from build123d import *

# Parameters (mm, degrees)
SKETCH2_W                      = 25.4
SKETCH2_H                      = 50.8
SKETCH2_W_2                    = 22.225
SKETCH2_H_2                    = 47.625
EXTRUDE_THIN2_DEPTH            = 1828.8
CUT_EXTRUDE1_DEPTH             = 26.4
F_9_16_0_5625_DIAMETER_HOLE1_D = 14.2875
F_9_16_0_5625_DIAMETER_HOLE2_D = 14.2875
F_12_0MM_DOWEL_HOLE1_D         = 12
F_3_16_0_1875_DIAMETER_HOLE1_D = 4.7625


with BuildPart() as part:
    # Sketch2 → Extrude-Thin2 (new body)
    with BuildSketch(Plane.XY):
        Rectangle(SKETCH2_W, SKETCH2_H)
        Rectangle(SKETCH2_W_2, SKETCH2_H_2, mode=Mode.SUBTRACT)
    extrude(amount=EXTRUDE_THIN2_DEPTH)

    # Sketch8 → Cut-Extrude1 (cut, through all)
    with BuildSketch(Plane(origin=(12.7, 0, 0), x_dir=(0, 0, -1), z_dir=(1, 0, 0))):
        with BuildLine():
            Line((-1828.8, 25.4), (-1828.8, -3.09e-07))
            ThreePointArc((-1828.8, -3.09e-07), (-1824.623790622, 14.87379041), (-1813.315860361, 25.4))
            Line((-1813.315860361, 25.4), (-1828.8, 25.4))
        make_face()
        with BuildLine():
            Line((-1828.8, -25.4), (-1813.315860361, -25.4))
            ThreePointArc((-1813.315860361, -25.4), (-1824.623790462, -14.873790674), (-1828.8, -3.09e-07))
            Line((-1828.8, -3.09e-07), (-1828.8, -25.4))
        make_face()
    extrude(amount=-CUT_EXTRUDE1_DEPTH, mode=Mode.SUBTRACT)

    # 9/16 (0.5625) Diameter Hole1 (through all)
    with Locations(Plane(origin=(12.7, 0, 0), x_dir=(0, 0, -1), z_dir=(1, 0, 0))):
        with Locations((-1800.225, 0)):
            Hole(F_9_16_0_5625_DIAMETER_HOLE1_D / 2)

    # 9/16 (0.5625) Diameter Hole2 (through all)
    with Locations(Plane(origin=(12.7, 0, 0), x_dir=(0, 0, -1), z_dir=(1, 0, 0))):
        with Locations((-542.925, 0)):
            Hole(F_9_16_0_5625_DIAMETER_HOLE2_D / 2)

    # Ø12.0mm Dowel Hole1 (through all)
    with Locations(Plane(origin=(12.7, 0, 0), x_dir=(0, 0, -1), z_dir=(1, 0, 0))):
        with Locations((-587.9703125, 0), (-497.8796875, 0)):
            Hole(F_12_0MM_DOWEL_HOLE1_D / 2)

    # 3/16 (0.1875) Diameter Hole1 (through all)
    with Locations(Plane(origin=(12.7, 0, 0), x_dir=(0, 0, -1), z_dir=(1, 0, 0))):
        with Locations((-1784.509551788, 15.715448212), (-1784.509551788, -15.715448212), (-1815.940448212, -15.715448212), (-1815.940448212, 15.715448212)):
            Hole(F_3_16_0_1875_DIAMETER_HOLE1_D / 2)


solid = part.part
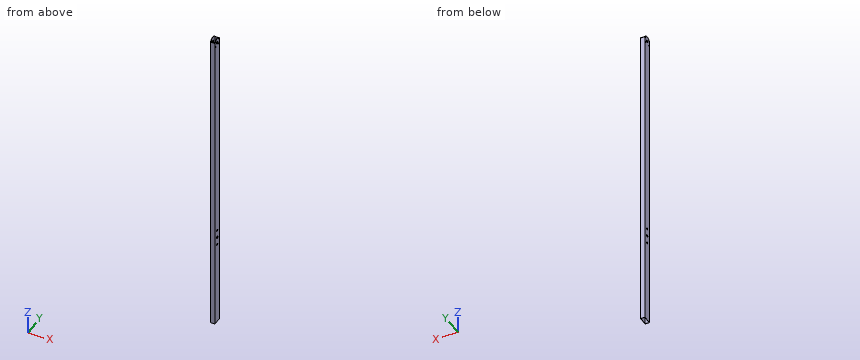
Can you work these out from the model? Positions are in its coordinate system, mm. Round coordinates to 2 decimals unless told otherwise and drop trailing zeros. Loops run counter-clockwise (first coordinate to the right, second up) from the corner with the lowest first, then second, coordinate; pieces in that order, holes last. Notation, with made-up numbers: (19, -23.5) - (36, -23.5) arc R30 ccw to (36, 6.5) - close; hole circle Ø5 at (24.5, -32.75). An arc over 180 degrees is marked (long way). Answer in a Markdown table with one row per item. Add a question column.
Q1. I need wall thicknesses on L1, parallel to X at y = 18.5, z = 1163; L2, parallel to Y at x = 2.25, z = 335. Which ranges of each line are inside material? Lowest first, please.
Q2. For pin 1 Ø12 at (x, y) = (6, 10) entering from +Z, with a flat end and sliding along its axis, tell me the tip position at first contact or that it passes through.
Q3. I want a section at B-B on z = 377. List the corners of the cut face in (x, y) for me, and give its area (3 significant figures).
A:
| question | item | result |
|---|---|---|
| 1 | L1 | -12.7 to -11.11, 11.11 to 12.7 |
| 1 | L2 | -25.4 to -23.81, 23.81 to 25.4 |
| 2 | pin 1 | z = 1827.96 |
| 3 | outline | (-12.7, -25.4) - (12.7, -25.4) - (12.7, 25.4) - (-12.7, 25.4) - close; hole (-11.11, -23.81) - (11.11, -23.81) - (11.11, 23.81) - (-11.11, 23.81) - close |
| 3 | area | 232 mm^2 |
